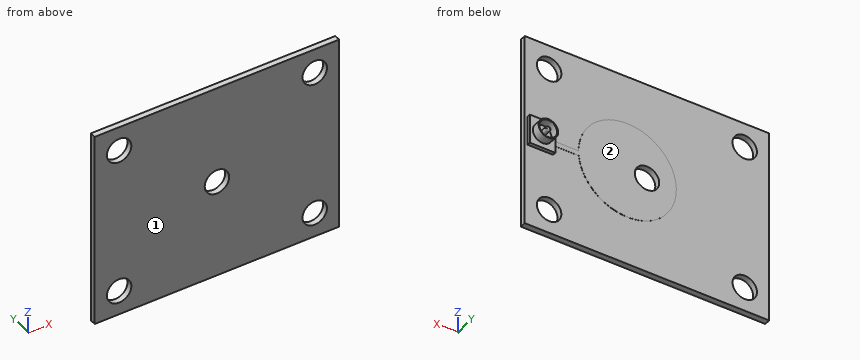
```python
from build123d import *

# Parameters (mm, degrees)
SKETCH1_W           = 25
SKETCH1_H           = 20
BOSS_EXTRUDE1_DEPTH = 0.6
SKETCH2_R           = 1.25
CUT_EXTRUDE1_DEPTH  = 0.6
SKETCH4_W           = 2.6
SKETCH4_H           = 3
BOSS_EXTRUDE2_DEPTH = 0.35
SKETCH5_R           = 1
BOSS_EXTRUDE3_DEPTH = 0.9
SKETCH6_R           = 0.9
SKETCH6_R_2         = 0.25
CUT_EXTRUDE2_DEPTH  = 0.9
FILLET1_R           = 0.1
FILLET2_R           = 0.05
BOSS_EXTRUDE9_START = 0.01
SKETCH8_R           = 1.25
BOSS_EXTRUDE9_DEPTH = 0.01


with BuildPart() as part:
    # Sketch1 → Boss-Extrude1 (new body)
    with BuildSketch(Plane(origin=(0, 0, 0), x_dir=(1, 0, 0), z_dir=(0, 1, 0))):
        Rectangle(SKETCH1_W, SKETCH1_H)
    extrude(amount=BOSS_EXTRUDE1_DEPTH)

    # Sketch2 → Cut-Extrude1 (cut)
    with BuildSketch(Plane(origin=(0, 0.6, 0), x_dir=(1, 0, 0), z_dir=(0, 1, 0))):
        with Locations(Location((-10, 7.5, 0), (0, 0, 270))):
            Circle(SKETCH2_R)
        with Locations(Location((10, 7.5, 0), (0, 0, 90))):
            Circle(SKETCH2_R)
        with Locations(Location((10, -7.5, 0), (0, 0, 270))):
            Circle(SKETCH2_R)
        with Locations(Location((-10, -7.5, 0), (0, 0, 90))):
            Circle(SKETCH2_R)
        with Locations(Location((0, 0, 0), (0, 0, 270))):
            Circle(SKETCH2_R)
    extrude(amount=-CUT_EXTRUDE1_DEPTH, mode=Mode.SUBTRACT)

    # Sketch4 → Boss-Extrude2 (add)
    with BuildSketch(Plane(origin=(0, 0.6, 0), x_dir=(1, 0, 0), z_dir=(0, 1, 0))):
        with Locations((10.9, 0)):
            Rectangle(SKETCH4_W, SKETCH4_H)
    extrude(amount=BOSS_EXTRUDE2_DEPTH)

    # Sketch5 → Boss-Extrude3 (add)
    with BuildSketch(Plane(origin=(0, 0.95, 0), x_dir=(1, 0, 0), z_dir=(0, 1, 0))):
        with Locations(Location((10.9, 0, 0), (0, 0, 270))):
            Circle(SKETCH5_R)
    extrude(amount=BOSS_EXTRUDE3_DEPTH)

    # Sketch6 → Cut-Extrude2 (cut)
    with BuildSketch(Plane(origin=(0, 1.85, 0), x_dir=(1, 0, 0), z_dir=(0, 1, 0))):
        with Locations(Location((10.9, 0, 0), (0, 0, 270))):
            Circle(SKETCH6_R)
        with Locations(Location((10.9, 0, 0), (0, 0, 270))):
            Circle(SKETCH6_R_2, mode=Mode.SUBTRACT)
    extrude(amount=-CUT_EXTRUDE2_DEPTH, mode=Mode.SUBTRACT)

    # Fillet1
    fillet1_edges = [part.edges().sort_by_distance(p)[0] for p in [
        (10.9, 1.85, -0.25),
    ]]
    fillet(fillet1_edges, radius=FILLET1_R)

    # Fillet2
    fillet2_edges = [part.edges().sort_by_distance(p)[0] for p in [
        (10.9, 1.85, -0.9),
    ]]
    fillet(fillet2_edges, radius=FILLET2_R)

    # Sketch8 → Boss-Extrude9 (add)
    # profile 1 of 3: a face of its own
    with BuildSketch(Plane(origin=(0, 0.6, 0), x_dir=(1, 0, 0), z_dir=(0, 1, 0)).offset(BOSS_EXTRUDE9_START)):
        with BuildLine():
            Line((6.991, -0.29986497), (7, 0))
            Line((7, 0), (1.25, 0))
            Line((1.25, 0), (1.25, 0.5))
            Line((1.25, 0.5), (6.974937186, 0.5))
            ThreePointArc((6.974937186, 0.5), (-2.998992097, -0.100389298), (6.991, -0.29986497))
        make_face()
        with Locations(Location((0, 0, 0), (0, 0, 270))):
            Circle(SKETCH8_R, mode=Mode.SUBTRACT)
    # profile 2 of 3: a face of its own
    with BuildSketch(Plane(origin=(0, 0.6, 0), x_dir=(1, 0, 0), z_dir=(0, 1, 0)).offset(BOSS_EXTRUDE9_START)):
        with BuildLine():
            Line((1.25, 0), (7, 0))
            ThreePointArc((7, 0), (6.993730366, 0.250313875), (6.974937186, 0.5))
            Line((6.974937186, 0.5), (1.25, 0.5))
            Line((1.25, 0.5), (1.25, 0))
        make_face()
    # profile 3 of 3: a face of its own
    with BuildSketch(Plane(origin=(0, 0.6, 0), x_dir=(1, 0, 0), z_dir=(0, 1, 0)).offset(BOSS_EXTRUDE9_START)):
        with BuildLine():
            ThreePointArc((6.974937186, 0.5), (6.993730366, 0.250313875), (7, 0))
            Line((7, 0), (9.6, 0))
            Line((9.6, 0), (9.6, 0.5))
            Line((9.6, 0.5), (6.974937186, 0.5))
        make_face()
    extrude(amount=-BOSS_EXTRUDE9_DEPTH)


solid = part.part
```
The model under review builds one solid part; all positions refer to its coordinate system, in mm. Face numbers are marked on the shaded views. A direction names the side the tool comes from. Coordinates: 2 decimals unless noted, no trailing zeros. Write each loop counter-clockwise with the first axis right and the second up, starting at its lowest first coordinate (ties: lowest second). Pieces come first, ordered by that corner, then holes. Notation, with made-up numbers: (72.25, -19.5) - (131.25, -19.5) arc R21 ccw to (131.25, 10.5) - close; hole circle Ø5 at (-32, -29.5). An arc over 180 degrees is marked (long way). Write item = value, one per line.
(1) For P1, Ø3, axis at x = -7, z = 5, coming from the +Y side; P2, Ø2, axis at x = 10, z = 7.5, coming from the -Y side, all flat-tipped, find the tip position at first contact; note any pin that passes through.
Result sheet:
P1 = 0.6
P2 = through
(2) Consider section A-A, the plane x = -10. Give the boundary of the cut face in (y, z), then the cut area to 3 significant figures.
Result sheet:
outline = (0, -10) - (0.6, -10) - (0.6, -8.75) - (0, -8.75) - close; (0, -6.25) - (0.6, -6.25) - (0.6, 6.25) - (0, 6.25) - close; (0, 8.75) - (0.6, 8.75) - (0.6, 10) - (0, 10) - close
area = 9.00 mm^2
(3) For line 1 (X direction, y = 0.3, z = 7.5); line 2 (X direction, y = 0.4, z = -8); line 3 (Y direction, x = -2.25, z = 9), list the stretches that pass through material, from the lowest coordinate up. Write a range as [from, to].
Result sheet:
line_1 = [-12.5, -11.25], [-8.75, 8.75], [11.25, 12.5]
line_2 = [-12.5, -11.15], [-8.85, 8.85], [11.15, 12.5]
line_3 = [0, 0.6]
(4) Consider section B-B, the plane z = -7.5. Give the boundary of the cut face in (x, y).
Result sheet:
outline = (-12.5, 0) - (-11.25, 0) - (-11.25, 0.6) - (-12.5, 0.6) - close; (-8.75, 0) - (8.75, 0) - (8.75, 0.6) - (-8.75, 0.6) - close; (11.25, 0) - (12.5, 0) - (12.5, 0.6) - (11.25, 0.6) - close
(5) Machinability: for the marked faces 1 and 2, which of the approach directions +Z, -Z, +X, -X, +Y, -Y give a long, thin tool a straight path to every point of the face, cutting with its end or side? Answer none if there is none.
Result sheet:
face_1 = +Z, -Z, +X, -X, -Y
face_2 = +Z, -Z, -X, +Y
